Geometry: see drawing. Coordinates: mm, zero at the bounding-box minimum. A direction names the side the tool comes from. Round coordinates to 2 decimals unless told otherwise and drop trailing zeros. Loops run counter-clockwise (first coordinate to the right, second up) from the corner with the lowest first, then second, coordinate; pieces in that order, holes last.
(1) Cut plane C-C, the plane z = 15. Output: boundary loops of the cut face in (x, y) (1 decimal).
(2) Line query: line 1 (Z direction, x = 7.75, y = 9.5); line 2 (X direction, y = 5.5, z = 5.5) (1 decimal). Output: solid intervals per line, ascending.
(3) Access query for the marked faces 1, 2 and 3. Directions: +Z, -Z, +X, -X, +Y, -Y. A direction counts if a zero-diameter tool reaches every point of the face in a straight line with its end or side. Return the directions, or none.
(4) Cut plane A-A, the plane x = 4.25. Output: boundary loops of the cut face in (y, z) (1 decimal).
(5) First-contact query: pin 1 Ø6 at (x, z) = (9, 3) entering from +Y; pin 2 Ø2 at (y, z) = (2.5, 17) entering from +X; pin 3 Ø1 at (x, z) = (3, 11) entering from -Y (1 decimal); pin 4 Ø3 at (x, y) = (7.5, 6) entering from -Z. Flat tips, straight axial feed; report the tip coordinate or a pass-through.
(6) Cut plane D-D, the plane z = 2.75. Output: boundary loops of the cut face in (x, y), and give its area (3 significant figures).
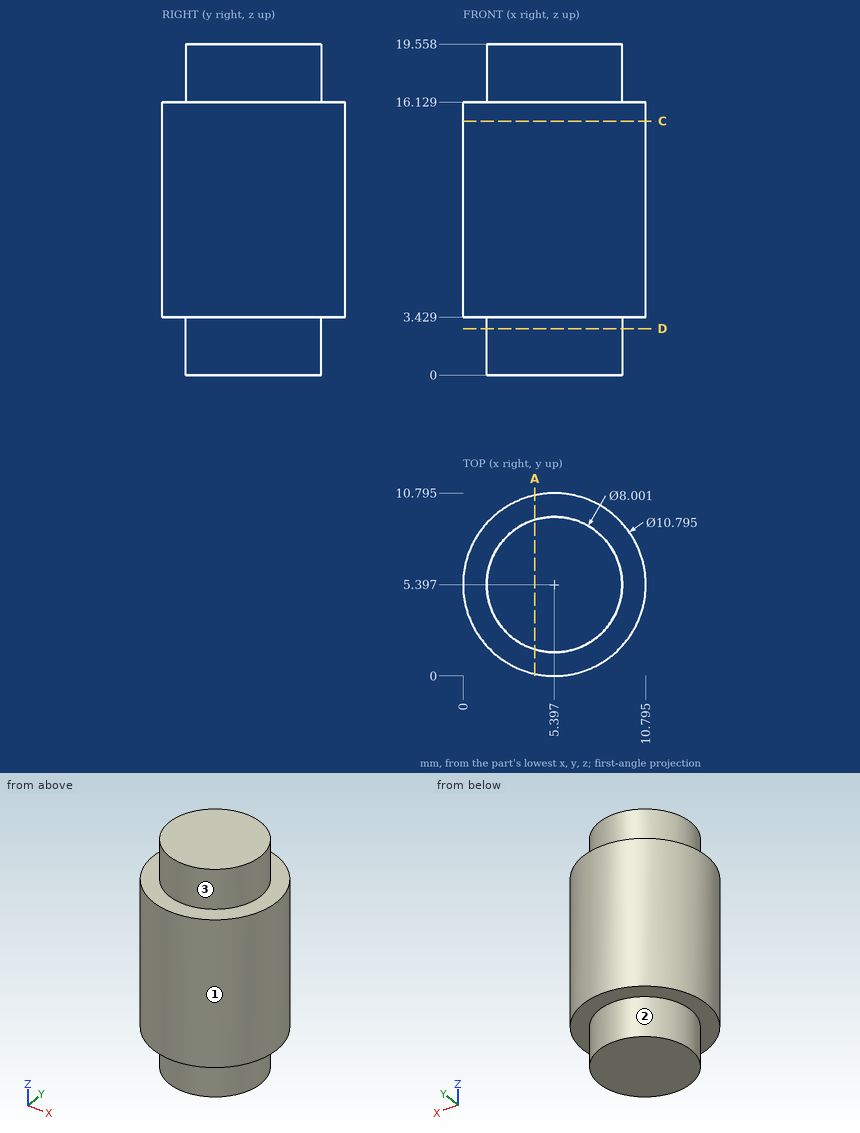
Reported:
1. outline: circle Ø10.8 at (5.4, 5.4)
2. line 1: z = 3.43 to 16.13
2. line 2: x = 0 to 10.8
3. face 1: +Z, -Z
3. face 2: -Z
3. face 3: +Z
4. outline: (0.1, 3.4) - (1.6, 3.4) - (1.6, 0) - (9.2, 0) - (9.2, 3.4) - (10.7, 3.4) - (10.7, 16.1) - (9.2, 16.1) - (9.2, 19.6) - (1.6, 19.6) - (1.6, 16.1) - (0.1, 16.1) - close
5. pin 1: stops at y = 10.76
5. pin 2: stops at x = 10.23
5. pin 3: stops at y = 0.3
5. pin 4: stops at z = 0
6. outline: circle Ø8 at (5.4, 5.4)
6. area: 50.3 mm2
